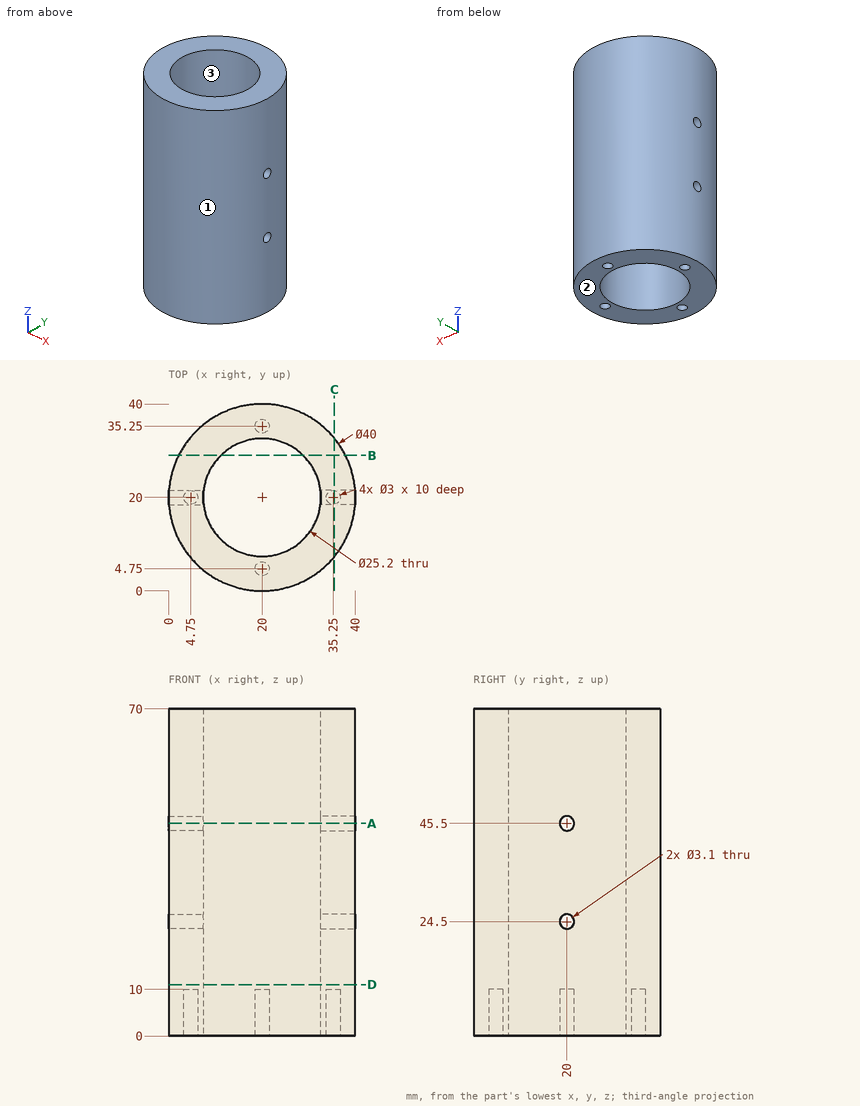
For this review, use the dimensioned drawing (mm, ordinates from the lowest corner) and the shaded views. Round coordinates to 2 decimals unless told otherwise and drop trailing zeros. Order: outer loops, then holes, each group sorted by start corner. A loop starts at its lowest first (then second) coordinate and runs counter-clockwise, first axis right, second up. Notation, with made-up numbers: (-4.5, -32.75) -> (38.5, -32.75) arc R30 cw to (38.5, 0.25) -> close; hole circle Ø5 at (78.5, -0.5). An arc over 180 degrees is marked (long way). One line per item, written item: value. Start each with the question number.
Q1. Take a section at B-B (y = 29). Write out the cut boundary in (x, z), and give its area (3 significant figures).
Q2. Wall thickness on line 1 (Z direction, x = 33.5, y = 19); line 2 (Y direction, x = 20, z = 43); line 3 (X direction, y = 10.5, z = 61.5): over which ranges is each line inside the solid? List them lowest first.
Q3. Mouldability with a two-part tool opening along X and no side actions: class the marked faces 1, 2 and 3 as released by +X, released by -X, zero draft, split by the parting line, or undercut.
Q4. Take a section at C-C (x = 35.5). Write out the cut boundary in (y, z), and give its area (3 significant figures).
Q5. Take a section at D-D (z = 11). Write out the cut boundary in (x, y).
Q6. Clearance check with flat-ended pins moving along their axes: pin 1 Ø1 at (x, z) = (30.5, 31) entering from +Y; pin 2 Ø6 at (y, z) = (15.5, 52) entering from +X; pin 3 Ø3 at (y, z) = (14.5, 26) entering from -X. State where each tip first meets the part, or that it passes through.
Q7. Take a section at A-A (z = 45.5). Write out the cut boundary in (x, y).
Reported:
1. outline: (2.14, 0) -> (11.18, 0) -> (11.18, 70) -> (2.14, 70) -> close; (28.82, 0) -> (37.86, 0) -> (37.86, 70) -> (28.82, 70) -> close
1. area: 1,270 mm2
2. line 1: z = 0 to 23.32, 25.68 to 44.32, 46.68 to 70
2. line 2: y = 0 to 7.4, 32.6 to 40
2. line 3: x = 2.4 to 11.72, 28.28 to 37.6
3. face 1: split by the parting line
3. face 2: zero draft
3. face 3: undercut
4. outline: (7.36, 0) -> (18.52, 0) -> (18.52, 10) -> (21.48, 10) -> (21.48, 0) -> (32.64, 0) -> (32.64, 70) -> (7.36, 70) -> close; hole circle Ø3.1 at (20, 24.5); hole circle Ø3.1 at (20, 45.5)
4. area: 1,720 mm2
5. outline: circle Ø40 at (20, 20); hole circle Ø25.2 at (20, 20)
6. pin 1: stops at y = 37.32
6. pin 2: stops at x = 39.94
6. pin 3: stops at x = 0.4
7. outline: (0.06, 18.45) arc R20 ccw to (39.94, 18.45) -> (32.5, 18.45) arc R12.6 cw to (7.5, 18.45) -> close; (0.06, 21.55) -> (7.5, 21.55) arc R12.6 cw to (32.5, 21.55) -> (39.94, 21.55) arc R20 ccw to start
